The listing builds one solid part. Answer for the finished solid, in the listing's coordinates (mm). Round coordinates to 2 decimals unless told otherwise and drop trailing zeros. Write each loop counter-clockwise with the first axis right and the second up, starting at its lowest first coordinate (ties: lowest second). Pieces come first, ordered by that corner, then holes. Notation, with made-up numbers: M 87,52.25 L 118,52.25 A27 cw 118,73.25 Z; hole C 67,-22.5 d4. An arc over 180 degrees is marked long. Write each question's results on one line, items separated by ' | '.
from build123d import *

# Parameters (mm, degrees)
CROQUIS1_R              = 2.34375
CROQUIS1_R_2            = 1
SALIENTE_EXTRUIR4_DEPTH = 5


with BuildPart() as part:
    # Croquis1 → Saliente-Extruir4 (new body)
    with BuildSketch(Plane.XY):
        with BuildLine():
            Line((0, 60), (0, 0))
            Line((0, 0), (33, 0))
            Line((33, 0), (33, 50))
            ThreePointArc((33, 50), (30.071067812, 57.071067812), (23, 60))
            Line((23, 60), (0, 60))
        make_face()
        with Locations((23, 50)):
            Circle(CROQUIS1_R, mode=Mode.SUBTRACT)
        with Locations((8, 5)):
            Circle(CROQUIS1_R_2, mode=Mode.SUBTRACT)
        with Locations((8, 35)):
            Circle(CROQUIS1_R_2, mode=Mode.SUBTRACT)
    extrude(amount=SALIENTE_EXTRUIR4_DEPTH)


solid = part.part
1) Section D-D (x = 21.5) is taken. Determine the outline of the cut face in (y, z).
Return value:
outline: M 0,0 L 48.2,0 L 48.2,5 L 0,5 Z; M 51.8,0 L 60,0 L 60,5 L 51.8,5 Z
2) Find the intervals of material crossed by line 1 (Y direction, x = 8, z = 3.5); line 2 (Y direction, x = 23, z = 2.9); line 3 (X direction, y = 51, z = 3.3), in increasing order.
Return value:
line 1: 0 to 4, 6 to 34, 36 to 60 | line 2: 0 to 47.66, 52.34 to 60 | line 3: 0 to 20.88, 25.12 to 32.95
3) The mould has two halves that part along X. Classify faces 1 (the face through (7.263, 5.676, 2.465)), 2 (the face through (0, 30, 2)), 3 (the face through (16, 30, 0)), 4 (the face through (30.15, 56.99, 2.46)): +X half, -X half, draft (parallel to the pull), parting line (faces both ways), or undercut.
Return value:
face 1: undercut | face 2: -X half | face 3: draft | face 4: +X half
4) Section B-B (z = 2.1) is taken. Determine the outline of the cut face in (x, y).
Return value:
outline: M 0,0 L 33,0 L 33,50 A10 ccw 23,60 L 0,60 Z; hole C 8,5 d2; hole C 8,35 d2; hole C 23,50 d4.69
5) Section A-A (y = 5) is taken. Determine the outline of the cut face in (x, z), then the cut area to 3 significant figures.
Return value:
outline: M 0,0 L 7,0 L 7,5 L 0,5 Z; M 9,0 L 33,0 L 33,5 L 9,5 Z | area: 155 mm²
6) Section C-C (x = 8) is taken. Determine the outline of the cut face in (y, z).
Return value:
outline: M 0,0 L 4,0 L 4,5 L 0,5 Z; M 6,0 L 34,0 L 34,5 L 6,5 Z; M 36,0 L 60,0 L 60,5 L 36,5 Z
